Check sheet for the drawn part. Datum: minimum x, y, z corner. Units: mm. Coordinates: 2 decimals unless noted, no trailing zeros. Order: outer loops, then holes, each group sorted by start corner. A loop starts at its lowest first (then second) coordinate and runs counter-clockwise, first axis right, second up.
Q1. Draft check along Y on the marked faces 1, 2 and 3. Enter one of: pulls with the +Y half, pulls with the -Y half, needs draft (parallel to the pull), parting line crosses it, or undercut.
Q2. Depth check by flat-ended pin: P1, Ø3, axis at x = 9.5, y = 9.5, coming from the +Z side; P2, Ø8, axis at y = 16.5, z = 9, coming from the -X side; P3, Ø1, axis at x = 2.5, y = 16, coming from the +Z side. Enter the tip coordinate at first touch or a pass-through.
Q3. Cross-section at D-D, the plane z = 19.5. Record the boundary of the cut face in (x, y), and give its area (3 significant figures).
Q4. Cross-section at A-A, the plane y = 9.5. Record the boundary of the cut face in (x, z).
Q5. Thickness scan on line 1 (Y direction, x = 9.5, z = 11); line 2 (Y direction, x = 9.5, z = 22.5); line 3 (X direction, y = 9, z = 6.25). Record the ranges inside material, lowest first.
Q6. Cross-section at C-C, the plane z = 9. Record the boundary of the cut face in (x, y).
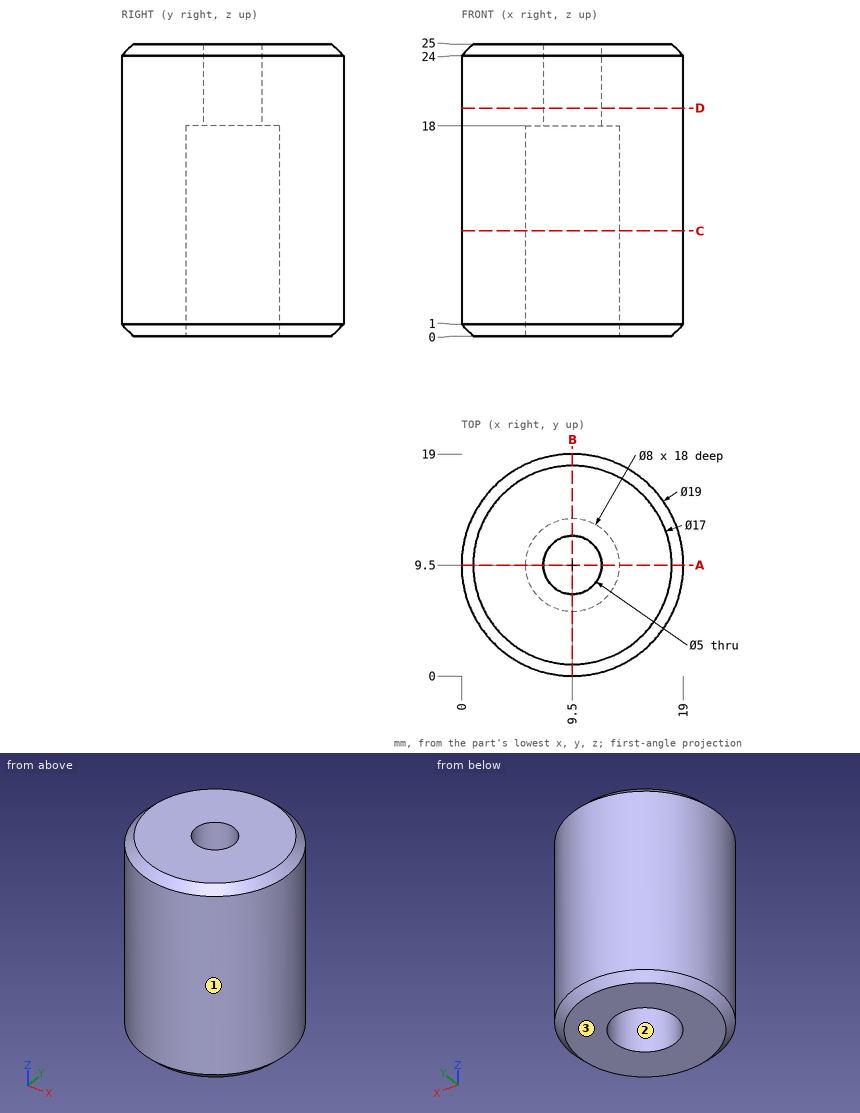
Check values:
1. face 1: parting line crosses it
1. face 2: undercut
1. face 3: needs draft
2. P1: passes through
2. P2: stops at x = 0.49
2. P3: stops at z = 24.45
3. outline: circle Ø19 at (9.5, 9.5); hole circle Ø5 at (9.5, 9.5)
3. area: 264 mm2
4. outline: (0, 1) - (1, 0) - (5.5, 0) - (5.5, 18) - (7, 18) - (7, 25) - (1, 25) - (0, 24) - close; (12, 18) - (13.5, 18) - (13.5, 0) - (18, 0) - (19, 1) - (19, 24) - (18, 25) - (12, 25) - close
5. line 1: y = 0 to 5.5, 13.5 to 19
5. line 2: y = 0 to 7, 12 to 19
5. line 3: x = 0.01 to 5.53, 13.47 to 18.99
6. outline: circle Ø19 at (9.5, 9.5); hole circle Ø8 at (9.5, 9.5)
